Verification items for the finished model (mm, model axes). Face numbers are marked on the shaded views. A direction names the side the tool comes from. Coordinates: 2 decimals unless noted, no trailing zeros. Loops run counter-clockwise (first coordinate to the right, second up) from the corner with the lowest first, then second, coordinate; pieces in that order, holes last. Notation, with made-up numbers: (-25.75, 66.5) - (-5.75, 66.5) arc R25 ccw to (-5.75, 96.5) - close; hole circle Ø11 at (16.25, 30.5). An arc over 180 degrees is marked (long way). One line per item, written item: value. Start each with the question number.
(1) Section check C-C (y = 10.75). Record the boundary of the cut face in (x, z).
(2) Section check D-D (x = 57.5). Record the boundary of the cut face in (y, z).
(3) Section check A-A (x = 0). Record the boundary of the cut face in (y, z), plus the area to 4 significant figures.
(4) Gauge pin test, flat ends, axial feed: P1, Ø8, axis at x = 0, z = 0, coming from the +Y side; P2, Ø3.5, axis at x = 35, y = 6.35, coming from the +Z side. Record the tip position at first contact, or that the pin passes through.
(5) Thickness scan on probe 1 along X at (y, z) = (10.5, 0); probe 2 along X at (y, z) = (6.35, 22); probe 3 along Z at (x, y) = (66.5, 5). Record the ranges inside material, lowest first. Write a range as [from, to].
(6) Set-up check for the marked faces 1 and 2: record each of +Z, -Z, +X, -X, +Y, -Y from which the full face is reachable in a straight line by a thin tool's end or side.
(7) Section check B-B (z = 0). Record the boundary of the cut face in (x, y).
(8) Draft check along X on the marked faces 3, 4 and 5. Enter one of: +X half, -X half, draft (parallel to the pull), parting line (faces both ways), or undercut.
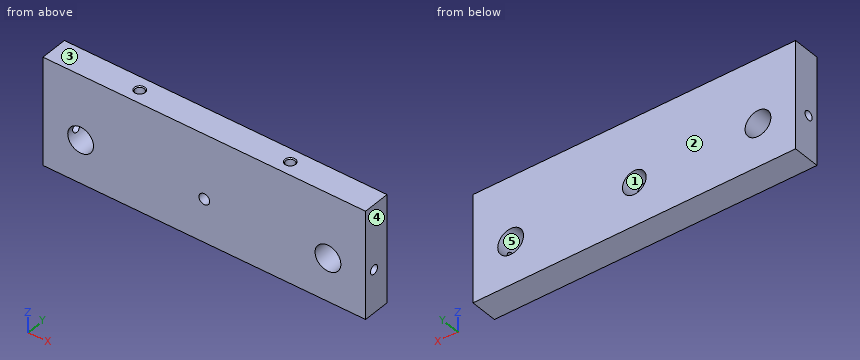
```python
from build123d import *

# Parameters (mm, degrees)
ESBO_O1_W                       = 150
ESBO_O1_H                       = 40
ESBO_O1_R                       = 2.5
RESSALTO_EXTRUS_O1_DEPTH        = 12.7
ESBO_O2_R                       = 5.5
CORTE_EXTRUS_O1_DEPTH           = 8
ESBO_O3_R                       = 6
CORTE_EXTRUS_O3_DEPTH           = 79.652971972
ESBO_O7_W                       = 150
ESBO_O7_H                       = 10
RESSALTO_EXTRUS_O2_DEPTH        = 12.7
ESBO_O8_R                       = 2
CORTE_EXTRUS_O4_DEPTH           = 10
FURO_ROSCADO_DE_M54_D           = 4.2
FURO_ROSCADO_DE_M54_DEPTH       = 12.4
FURO_ROSCADO_DE_M54_CSINK_D     = 5.05
FURO_ROSCADO_DE_M54_CSINK_ANGLE = 90
FURO_ROSCADO_DE_M54_TIP         = 1.2618073
FURO_ROSCADO_DE_M55_D           = 4.2
FURO_ROSCADO_DE_M55_DEPTH       = 12.4
FURO_ROSCADO_DE_M55_CSINK_D     = 5.05
FURO_ROSCADO_DE_M55_CSINK_ANGLE = 90
FURO_ROSCADO_DE_M55_TIP         = 1.2618073


with BuildPart() as part:
    # Esboço1 → Ressalto-extrusão1 (new body)
    with BuildSketch(Plane(origin=(0, 0, 0), x_dir=(1, 0, 0), z_dir=(0, 1, 0))):
        Rectangle(ESBO_O1_W, ESBO_O1_H)
        with Locations(Location((0, 0, 0), (0, 0, 270))):
            Circle(ESBO_O1_R, mode=Mode.SUBTRACT)
    extrude(amount=RESSALTO_EXTRUS_O1_DEPTH)

    # Esboço2 → Corte-extrusão1 (cut)
    with BuildSketch(Plane(origin=(0, 12.7, 0), x_dir=(1, 0, 0), z_dir=(0, 1, 0))):
        with Locations(Location((0, 0, 0), (0, 0, 270))):
            Circle(ESBO_O2_R)
    extrude(amount=-CORTE_EXTRUS_O1_DEPTH, mode=Mode.SUBTRACT)

    # Esboço3 → Corte-extrusão3 (cut, through all)
    with BuildSketch(Plane(origin=(0, 12.7, 0), x_dir=(1, 0, 0), z_dir=(0, 1, 0))):
        with Locations(Location((-57.5, 0, 0), (0, 0, 270))):
            Circle(ESBO_O3_R)
        with Locations(Location((57.5, 0, 0), (0, 0, 270))):
            Circle(ESBO_O3_R)
    extrude(amount=-CORTE_EXTRUS_O3_DEPTH, mode=Mode.SUBTRACT)

    # Esboço6 → Furo roscado de M51 (revolve, cut)
    with BuildSketch(Plane(origin=(75, 5, 0), x_dir=(0, 0, -1), z_dir=(0, 1, 0))):
        Polygon((0, 0), (0, 13.2618073), (2.1, 12), (2.1, 0), align=None)
    furo_roscado_de_m51 = revolve(axis=Axis((81.35, 5, 0), (-1, 0, 0)), mode=Mode.SUBTRACT)

    # Espelhar1: Furo roscado de M51 across plane
    add(furo_roscado_de_m51.mirror(Plane(origin=(0, 0, 0), x_dir=(0, 0, 1), z_dir=(1, 0, 0))), mode=Mode.SUBTRACT)

    # Esboço7 → Ressalto-extrusão2 (add)
    with BuildSketch(Plane(origin=(0, 12.7, 0), x_dir=(1, 0, 0), z_dir=(0, 1, 0))):
        with Locations((0, -25)):
            Rectangle(ESBO_O7_W, ESBO_O7_H)
    extrude(amount=-RESSALTO_EXTRUS_O2_DEPTH)

    # Esboço8 → Corte-extrusão4 (cut)
    with BuildSketch(Plane.XY.offset(30)):
        with Locations((35, 6.35)):
            Circle(ESBO_O8_R)
        with Locations((-35, 6.35)):
            Circle(ESBO_O8_R)
    extrude(amount=-CORTE_EXTRUS_O4_DEPTH, mode=Mode.SUBTRACT)

    # Furo roscado de M54
    with Locations(Plane.XY.offset(30)):
        with Locations((-35, 6.35)):
            CounterSinkHole(FURO_ROSCADO_DE_M54_D / 2, FURO_ROSCADO_DE_M54_CSINK_D / 2, depth=FURO_ROSCADO_DE_M54_DEPTH, counter_sink_angle=FURO_ROSCADO_DE_M54_CSINK_ANGLE)
            with Locations((0, 0, -(FURO_ROSCADO_DE_M54_DEPTH + FURO_ROSCADO_DE_M54_TIP / 2))):  # 118° drill point
                Cone(0, FURO_ROSCADO_DE_M54_D / 2, FURO_ROSCADO_DE_M54_TIP, mode=Mode.SUBTRACT)

    # Furo roscado de M55
    with Locations(Plane.XY.offset(30)):
        with Locations((35, 6.35)):
            CounterSinkHole(FURO_ROSCADO_DE_M55_D / 2, FURO_ROSCADO_DE_M55_CSINK_D / 2, depth=FURO_ROSCADO_DE_M55_DEPTH, counter_sink_angle=FURO_ROSCADO_DE_M55_CSINK_ANGLE)
            with Locations((0, 0, -(FURO_ROSCADO_DE_M55_DEPTH + FURO_ROSCADO_DE_M55_TIP / 2))):  # 118° drill point
                Cone(0, FURO_ROSCADO_DE_M55_D / 2, FURO_ROSCADO_DE_M55_TIP, mode=Mode.SUBTRACT)


solid = part.part
```
Responses:
1. outline: (-75, -20) - (75, -20) - (75, 30) - (-75, 30) - close; hole circle Ø12 at (-57.5, 0); hole circle Ø11 at (0, 0); hole circle Ø12 at (57.5, 0)
2. outline: (0, -20) - (12.7, -20) - (12.7, -6) - (0, -6) - close; (0, 6) - (12.7, 6) - (12.7, 30) - (0, 30) - close
3. outline: (0, -20) - (12.7, -20) - (12.7, -5.5) - (4.7, -5.5) - (4.7, -2.5) - (0, -2.5) - close; (0, 2.5) - (4.7, 2.5) - (4.7, 5.5) - (12.7, 5.5) - (12.7, 30) - (0, 30) - close
3. area: 523.5 mm²
4. P1: stops at y = 4.7
4. P2: stops at z = 17.39
5. probe 1: x = [-75, -63.5], [-51.5, -5.5], [5.5, 51.5], [63.5, 75]
5. probe 2: x = [-75, -37.1], [-32.9, 32.9], [37.1, 75]
5. probe 3: z = [-20, -2.1], [2.1, 30]
6. face 1: +Y
6. face 2: +Z, -Z, +X, -X, +Y
7. outline: (-75, 0) - (-63.5, 0) - (-63.5, 2.9) - (-75, 2.9) - close; (-75, 7.1) - (-63.5, 7.1) - (-63.5, 12.7) - (-75, 12.7) - close; (-51.5, 0) - (-2.5, 0) - (-2.5, 4.7) - (-5.5, 4.7) - (-5.5, 12.7) - (-51.5, 12.7) - close; (2.5, 0) - (51.5, 0) - (51.5, 12.7) - (5.5, 12.7) - (5.5, 4.7) - (2.5, 4.7) - close; (63.5, 0) - (75, 0) - (75, 2.9) - (63.5, 2.9) - close; (63.5, 7.1) - (75, 7.1) - (75, 12.7) - (63.5, 12.7) - close
8. face 3: draft
8. face 4: +X half
8. face 5: undercut
